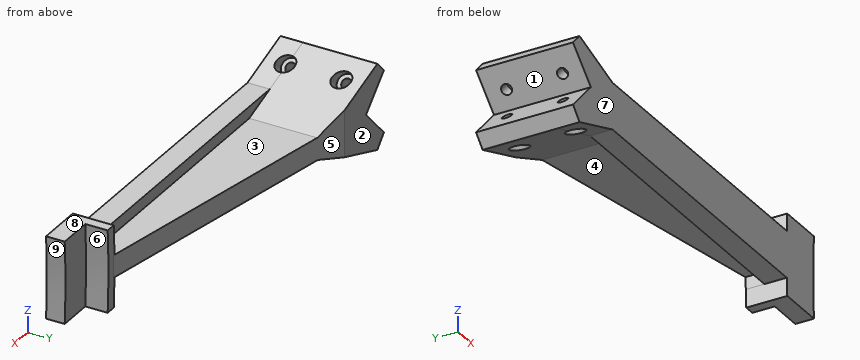
from build123d import *

# Parameters (mm, degrees)
BOSS_EXTRUDE2_DEPTH          = 12
BOSS_EXTRUDE3_START          = -2
BOSS_EXTRUDE3_DEPTH          = 10
BOSS_EXTRUDE4_START          = 10
BOSS_EXTRUDE4_DEPTH          = 22
BOSS_EXTRUDE7_DEPTH          = 40
BOSS_EXTRUDE17_DEPTH         = 6
BOSS_EXTRUDE17_DEPTH_BACK    = 6
CUT_EXTRUDE_THIN1_DEPTH      = 204.107832617
CUT_EXTRUDE_THIN1_DEPTH_BACK = 204.107832617
CUT_EXTRUDE1_START           = -8
SKETCH6_R                    = 5
CUT_EXTRUDE1_DEPTH           = 163.861994657
SKETCH6_4_R                  = 2.75
CUT_EXTRUDE2_DEPTH           = 171.861994657


with BuildPart() as part:
    # Sketch2 → Boss-Extrude2 (new body)
    with BuildSketch(Plane(origin=(0, 0, 0), x_dir=(1, 0, 0), z_dir=(0, 1, 0))):
        with BuildLine():
            Line((-197.696610314, 15.743442535), (-181.12456554, 0))
            Line((-181.12456554, 0), (-197.696610314, -17.444257657))
            Line((-197.696610314, -17.444257657), (-191.610767905, -23.850407561))
            Line((-191.610767905, -23.850407561), (-161.12456554, -12.777855375))
            Line((-161.12456554, -12.777855375), (0.21086679, -12.5))
            ThreePointArc((0.21086679, -12.5), (0.401744327, -17.25142014), (0.653571446, -22))
            Line((0.653571446, -22), (6.263616969, -22))
            ThreePointArc((6.263616969, -22), (5.6, 0), (6.263616969, 22))
            Line((6.263616969, 22), (0.653571446, 22))
            ThreePointArc((0.653571446, 22), (0.401744327, 17.25142014), (0.21086679, 12.5))
            Line((0.21086679, 12.5), (-161.12456554, 12.222144625))
            Line((-161.12456554, 12.222144625), (-191.610767905, 22.149592439))
            Line((-191.610767905, 22.149592439), (-197.696610314, 15.743442535))
        make_face()
    extrude(amount=-BOSS_EXTRUDE2_DEPTH)

    # Sketch2<5> → Boss-Extrude3 (add)
    with BuildSketch(Plane(origin=(0, 0, 0), x_dir=(1, 0, 0), z_dir=(0, 1, 0)).offset(BOSS_EXTRUDE3_START)):
        with BuildLine():
            Line((25.340211435, 22), (6.263616969, 22))
            ThreePointArc((6.263616969, 22), (5.6, 0), (6.263616969, -22))
            Line((6.263616969, -22), (25.340211435, -22))
            ThreePointArc((25.340211435, -22), (24.64, 0), (25.340211435, 22))
        make_face()
    extrude(amount=-BOSS_EXTRUDE3_DEPTH)

    # Sketch2<6> → Boss-Extrude4 (add)
    with BuildSketch(Plane(origin=(0, 0, 0), x_dir=(1, 0, 0), z_dir=(0, 1, 0)).offset(BOSS_EXTRUDE4_START)):
        with BuildLine():
            ThreePointArc((0.653571446, 22), (0.401744327, 17.25142014), (0.21086679, 12.5))
            ThreePointArc((0.21086679, 12.5), (0, 0), (0.21086679, -12.5))
            ThreePointArc((0.21086679, -12.5), (0.401744327, -17.25142014), (0.653571446, -22))
            Line((0.653571446, -22), (6.263616969, -22))
            ThreePointArc((6.263616969, -22), (5.6, 0), (6.263616969, 22))
            Line((6.263616969, 22), (0.653571446, 22))
        make_face()
    extrude(amount=-BOSS_EXTRUDE4_DEPTH)

    # Sketch2<9> → Boss-Extrude7 (add)
    with BuildSketch(Plane(origin=(0, 0, 0), x_dir=(1, 0, 0), z_dir=(0, 1, 0))):
        Polygon((-197.696610314, 15.743442535), (-181.12456554, 0), (-197.696610314, -17.444257657), (-191.610767905, -23.850407561), (-124.831467486, 0.40375437), (-191.610767905, 22.149592439), align=None)
    extrude(amount=BOSS_EXTRUDE7_DEPTH)

    # Sketch4 → Boss-Extrude17 (add, two sides: drawn at the far end of the back side and taken through both)
    with BuildSketch(Plane.XY.offset(-BOSS_EXTRUDE17_DEPTH_BACK)):
        Polygon((0.653571446, 10), (-161.12456554, 40), (-161.12456554, 0), (0.653571446, 0), align=None)
    extrude(amount=BOSS_EXTRUDE17_DEPTH + BOSS_EXTRUDE17_DEPTH_BACK)

    # Sketch5 → Cut-Extrude-Thin1 (cut, two sides: drawn at the far end of the back side and taken through both)
    with BuildSketch(Plane.XY.offset(-CUT_EXTRUDE_THIN1_DEPTH_BACK)):
        Polygon((0.653571446, 10), (-161.12456554, 40), (-159.301258723, 49.832372666), (2.476878263, 19.832372666), align=None)
    extrude(amount=CUT_EXTRUDE_THIN1_DEPTH + CUT_EXTRUDE_THIN1_DEPTH_BACK, mode=Mode.SUBTRACT)

    # Sketch6 → Cut-Extrude1 (cut, through all)
    with BuildSketch(Plane(origin=(-95.203451007, 0, -90.443278456), x_dir=(-0.6887494619146907, 0, 0.724999433594416), z_dir=(-0.724999433594416, 0, -0.6887494619146907)).offset(CUT_EXTRUDE1_START)):
        with Locations((134.749447055, 29)):
            Circle(SKETCH6_R)
        with Locations((134.749447055, -1)):
            Circle(SKETCH6_R)
    cut_extrude1 = extrude(amount=-CUT_EXTRUDE1_DEPTH, mode=Mode.SUBTRACT)

    # Sketch6<4> → Cut-Extrude2 (cut, symmetric)
    with BuildSketch(Plane(origin=(-95.203451007, 0, -90.443278456), x_dir=(-0.6887494619146907, 0, 0.724999433594416), z_dir=(-0.724999433594416, 0, -0.6887494619146907))):
        with Locations((134.749447055, 29)):
            Circle(SKETCH6_4_R)
        with Locations((134.749447055, -1)):
            Circle(SKETCH6_4_R)
    cut_extrude2 = extrude(amount=CUT_EXTRUDE2_DEPTH, both=True, mode=Mode.SUBTRACT)

    # Mirror1: Cut-Extrude1, Cut-Extrude2 across plane
    add(cut_extrude1.mirror(Plane.XY), mode=Mode.SUBTRACT)
    add(cut_extrude2.mirror(Plane.XY), mode=Mode.SUBTRACT)


with BuildPart() as body_2:
    # Mirror3: mirrored copy
    add(part.part.mirror(Plane.XY))


solid = body_2.part
For this review, take the finished solid that the model builds, in its own axes (mm). Face numbers are marked on the shaded views. A direction names the side the tool comes from. Round coordinates to 2 decimals unless told otherwise and drop trailing zeros. Loops run counter-clockwise (first coordinate to the right, second up) from the corner with the lowest first, then second, coordinate; pieces in that order, holes last. Notation, with made-up numbers: (30.25, 47) - (84.25, 47) arc R9 ccw to (84.25, 64) - close; hole circle Ø10 at (-7.5, 88.5). An arc over 180 degrees is marked (long way). One line per item, written item: value. Start each with the question number.
Item 1: For L1, parallel to Z at x = -94.5, y = 27.5; L2, parallel to Y at x = -90.5, z = -12; L3, parallel to Y at x = -142.5, z = 0.5, list the stretches that pass through material, from the lowest coordinate up.
Item 2: Clearance check with flat-ended pins moving along their axes: pin 1 Ø16 at (x, z) = (14, 4.5) entering from +Y; pin 2 Ø17.5 at (x, y) = (18.5, 1.5) entering from +Z; pin 3 Ø7 at (x, z) = (-110.5, 8) entering from +Y. State where each tip first meets the part, or that it passes through.
Item 3: Take a section at A-A (y = -8). Give the boundary of the cut face in (x, z), plus the area to 3 significant figures.
Item 4: Take a section at D-D (y = 20). Give the boundary of the cut face in (x, z).
Item 5: Take a section at B-B (x = -128). Give the boundary of the cut face in (y, z), plus the area to 3 significant figures.
Item 6: For the marked faces 1, 2, 3, 4 and 5, list the 3-axis set-ups (+Z, -Z, +X, -X, +Y, -Y) from which the entire face can be reached by the end or side of a thin tool; tool diameter is ignored.
Item 7: The part is to be moulded in two halves that separate along Z. For the marked faces 6, 7, 8 and 9, say which applies: +Z half, -Z half, draft (parallel to the pull), parting line (faces both ways), or undercut.
Item 8: Take a section at C-C (z = -2.5). Give the boundary of the cut face in (x, y).
Answer below:
1. L1: z = -6 to 6
1. L2: y = -12 to 0
1. L3: y = -12 to 36.55
2. pin 1: stops at y = -2
2. pin 2: stops at z = 22
2. pin 3: stops at y = 31.14
3. outline: (-197.7, -17.44) - (-191.61, -23.85) - (-161.12, -12.78) - (0.21, -12.5) arc R370.6 ccw to (0.65, -22) - (25.34, -22) arc R345.96 cw to (25.34, 22) - (0.65, 22) arc R370.6 ccw to (0.21, 12.5) - (-161.12, 12.22) - (-191.61, 22.15) - (-197.7, 15.74) - (-181.12, 0) - close
3. area: 6,160 mm2
4. outline: (-197.7, -17.44) - (-191.61, -23.85) - (-142.46, -6) - (-53.27, -6) - (-53.27, 6) - (-142.02, 6) - (-191.61, 22.15) - (-197.7, 15.74) - (-181.12, 0) - close
5. outline: (-12, -12.72) - (0, -12.72) - (0, -6) - (33.86, -6) - (33.86, 6) - (0, 6) - (0, 12.28) - (-12, 12.28) - close
5. area: 706 mm2
6. face 1: -X, +Y, -Y
6. face 2: +Z, -Z, +X, -X, +Y
6. face 3: +Z, +Y
6. face 4: -Z, +Y
6. face 5: +Z, -Z, +X, +Y
7. face 6: undercut
7. face 7: draft
7. face 8: +Z half
7. face 9: undercut
8. outline: (-183.5, -12) - (24.65, -12) - (24.65, -2) - (5.61, -2) - (5.61, 10) - (0.65, 10) - (-161.12, 40) - (-183.5, 40) - close
